Part model, mm, in its own coordinate system. A direction names the side the tool comes from. Give positions to 0.01 mm unless a question says otherwise; leave off trailing zeros. Order: outer loops, then holes, each group sorted by start corner. A loop starts at its lowest first (then second) coordinate and runs counter-clockwise, first axis right, second up. Notation, with made-up numbers: (49, 84.25) - (85, 84.25) arc R24 ccw to (85, 123.25) - close; hole circle Ø7 at (33, 6.5). An arc over 180 degrees is marked (long way). One line per item, written item: value.
Autodesk Inventor part; units mm, degrees
ref_plane "YZ Plane" through (0, 0, 0) normal (1, 0, 0) x (0, 1, 0)
ref_plane "XZ Plane" through (0, 0, 0) normal (0, 1, 0) x (-1, 0, 0)
ref_plane "XY Plane" through (0, 0, 0) normal (0, 0, 1) x (1, 0, 0)
sketch "Sketch1" plane through (0, 0, 0) normal (0, 0, 1) x (1, 0, 0)
  line L0 (3.7445, 22.5918) -> (94.5135, 7.547)
  line L1 (94.5135, -7.547) -> (3.7445, -22.5918)
  arc A0 (94.5135, -7.547) -> (94.5135, 7.547) centre (93.2626, 0) ccw
  arc A1 (3.7445, 22.5918) -> (3.7445, -22.5918) centre (0, 0) ccw
  line L2 (94.7211, 8.7999) -> (3.9522, 23.8447)
  arc A2 (3.9522, 23.8447) -> (3.9522, -23.8447) centre (0, 0) ccw
  line L3 (3.9522, -23.8447) -> (94.7211, -8.7999)
  arc A3 (94.7211, -8.7999) -> (94.7211, 8.7999) centre (93.2626, 0) ccw
  dimension "d7" = 1.27
extrude "Extrusion1" add sketch "Sketch1" along normal blind 9
ref_plane "Work Plane1" through (0, 0, 4.5) normal (0, 0, 1) x (1, 0, 0)
sketch "Sketch2" plane through (0, 0, 4.5) normal (0, 0, 1) x (1, 0, 0)
  arc A0 (3.7445, 22.5918) -> (3.7445, -22.5918) centre (0, 0) ccw
  line L0 (94.5135, 7.547) -> (3.7445, 22.5918)
  arc A1 (94.5135, -7.547) -> (94.5135, 7.547) centre (93.2626, 0) ccw
  line L1 (3.7445, -22.5918) -> (94.5135, -7.547)
  arc A2 (3.4995, 21.1133) -> (3.4995, -21.1133) centre (0, 0) ccw
  line L2 (3.4995, 21.1133) -> (94.2684, 6.0686)
  arc A3 (94.2684, -6.0686) -> (94.2684, 6.0686) centre (93.2626, 0) ccw
  line L3 (94.2684, -6.0686) -> (3.4995, -21.1133)
  dimension "d11" = 1.4986
extrude "Extrusion2" add sketch "Sketch2" along normal mid plane 8.9746
equation "\"d5\" = 45.8"
equation "\"d6\" = 15.3"
properties part number "285 mm Belt"
1) Drill centre lines: line 1 along X through (y, z) = (0.5, 3.5); line 2 along Y through (x, z) = (0, 6); line 3 along Y through (x, z) = (32, 2). Where is each one in solid material? Low to high. Write a range as from..to.
Outcome:
line 1: x = -24.16..-21.4, 99.39..102.17
line 2: y = -24.17..-21.4, 21.4..24.17
line 3: y = -19.2..-16.39, 16.39..19.2
2) Cut at C-C, the plane z = 5.5. Give the cut face in (x, y).
Outcome:
outline: (3.95, -23.84) - (94.72, -8.8) arc R8.92 ccw to (94.72, 8.8) - (3.95, 23.84) arc R24.17 ccw (long way) to start; hole (3.5, -21.11) - (94.27, -6.07) arc R6.15 ccw to (94.27, 6.07) - (3.5, 21.11) arc R21.4 ccw (long way) to start
3) Which spindle directions (+Z, -Z, +X, -X, +Y, -Y) get a long thin tool onto all of the face, cutting with end or side? Do faces 4 (the flat face through (34, -17, 0.013)), 5 (the cylindrical face through (99.413, 0.121, 4.437)). Say none if no direction does.
Outcome:
face 4: -Z, +X, -X, +Y, -Y
face 5: +Z, -Z
4) Mould opens along X. For faces 1 (the flat face through (34, 18, 0)), 2 (the flat face through (48.249, 13.696, 4.437)), 3 (the flat face through (48.701, -16.428, 4.437)) say: released by +X, released by -X, zero draft, split by the parting line, or undercut.
Outcome:
face 1: zero draft
face 2: undercut
face 3: released by +X
5) Pin check, flat tips, straight feed: pin 1 (5 mm diameter, centred on x = 44, z = 8, fed in from +Y); pin 2 (12 mm diameter, centred on x = 25, y = -14, fed in from +Z); pin 3 (1 mm diameter, centred on y = -16, z = 6, fed in from -X); pin 4 (5 mm diameter, centred on y = 13.5, z = 4, fed in from -X). Stop position of each tip, or through.
Outcome:
pin 1: stops at y = 17.62
pin 2: stops at z = 9
pin 3: stops at x = -18.55
pin 4: stops at x = -21.52
